from build123d import *

# Parameters (mm, degrees)
SKETCH1_R           = 15
BOSS_EXTRUDE1_DEPTH = 6
SKETCH2_R           = 30
BOSS_EXTRUDE2_DEPTH = 3
SKETCH5_R           = 10
CUT_EXTRUDE2_DEPTH  = 44.370496884
SKETCH8_R           = 2.5
CUT_EXTRUDE3_DEPTH  = 44.370496884


with BuildPart() as part:
    # Sketch1 → Boss-Extrude1 (new body)
    with BuildSketch(Plane.XY):
        Circle(SKETCH1_R)
    extrude(amount=BOSS_EXTRUDE1_DEPTH)

    # Sketch2 → Boss-Extrude2 (add)
    with BuildSketch(Plane.XY.offset(6)):
        Circle(SKETCH2_R)
    extrude(amount=BOSS_EXTRUDE2_DEPTH)

    # Sketch5 → Cut-Extrude2 (cut, through all)
    with BuildSketch(Plane(origin=(0, 0, 0), x_dir=(-1, 0, 0), z_dir=(0, 0, -1))):
        Circle(SKETCH5_R)
    extrude(amount=-CUT_EXTRUDE2_DEPTH, mode=Mode.SUBTRACT)

    # Sketch8 → Cut-Extrude3 (cut, through all)
    with BuildSketch(Plane.XY.offset(9)):
        with Locations((0, 25)):
            Circle(SKETCH8_R)
        with Locations((8.550503583, 23.49231552)):
            Circle(SKETCH8_R)
        with Locations((16.069690242, 19.151111078)):
            Circle(SKETCH8_R)
        with Locations((21.650635095, 12.5)):
            Circle(SKETCH8_R)
        with Locations((24.620193825, 4.341204442)):
            Circle(SKETCH8_R)
        with Locations((24.620193825, -4.341204442)):
            Circle(SKETCH8_R)
        with Locations((21.650635095, -12.5)):
            Circle(SKETCH8_R)
        with Locations((16.069690242, -19.151111078)):
            Circle(SKETCH8_R)
        with Locations((8.550503583, -23.49231552)):
            Circle(SKETCH8_R)
        with Locations((0, -25)):
            Circle(SKETCH8_R)
        with Locations((-8.550503583, -23.49231552)):
            Circle(SKETCH8_R)
        with Locations((-16.069690242, -19.151111078)):
            Circle(SKETCH8_R)
        with Locations((-21.650635095, -12.5)):
            Circle(SKETCH8_R)
        with Locations((-24.620193825, -4.341204442)):
            Circle(SKETCH8_R)
        with Locations((-24.620193825, 4.341204442)):
            Circle(SKETCH8_R)
        with Locations((-21.650635095, 12.5)):
            Circle(SKETCH8_R)
        with Locations((-16.069690242, 19.151111078)):
            Circle(SKETCH8_R)
        with Locations((-8.550503583, 23.49231552)):
            Circle(SKETCH8_R)
    extrude(amount=-CUT_EXTRUDE3_DEPTH, mode=Mode.SUBTRACT)


solid = part.part
Input: part model. Units: mm. Frame: model coordinates. A direction names the side the tool comes from. Give positions to 0.01 mm unless a question says otherwise; leave off trailing zeros. Loops run counter-clockwise (first coordinate to the right, second up) from the corner with the lowest first, then second, coordinate; pieces in that order, holes last. Notation, with made-up numbers: (-15.75, -28) -> (40.25, -28) arc R8 ccw to (40.25, -22) -> close; hole circle Ø6 at (45, 64.5). An arc over 180 degrees is marked (long way). Answer as a JSON object with one key per item and string values. Group by question number.
Item 1: Line query: probe 1 along X at (y, z) = (-20, 7.5); probe 2 along Y at (x, z) = (10.5, 8); probe 3 along Y at (x, z) = (0, 6.8). Output: solid intervals per line, ascending.
Item 2: Pin query (flat end, axial travel): P1, Ø5, axis at x = 10.5, z = 2.5, coming from the +Y side; P2, Ø4, axis at x = -24.62, y = -4.34, coming from the -Z side; P3, Ø6, axis at x = -8.55, y = 23.49, coming from the -Z side; P4, Ø1.5, axis at y = -12.5, z = 3.5, coming from the -X side. Return the tip coordinate at first contact, or that it passes through.
Item 3: Cut plane D-D, the plane z = 3.75. Return the cut outline in (x, y), and give its area (3 significant figures).
Item 4: Cut plane B-B, the plane y = 0. Return the cut outline in (x, z).
Item 5: Cut plane C-C, the plane x = -17.5. Return the cut outline in (y, z), and give its area (3 significant figures).
Item 6: Reachability of faces 4 (the cylindrical face through (-16.61, -21.59, 7.52)), 5 (the flat face through (6, 14, 6)) from +Z, -Z, +X, -X, +Y, -Y: full face, straight path, thin tool, end or side. Return the list, or none.
Item 7: Pull-direction query (Y, two-part tool) for faces 1 (the cylindrical face through (26.93, 3.38, 7.52)), 2 (the flat face through (13, 0, 9)), 3 (the cylindrical face through (-29.97, 1.32, 7.48)); classes: released by +Y, released by -Y, zero draft, split by the parting line, or undercut.
Item 8: Cut plane A-A, the plane x = 0. Return the cut outline in (y, z).
Checks:
{
 "1": {"probe 1": "x = -22.36 to -18.42, -13.72 to 13.72, 18.42 to 22.36", "probe 2": "y = -28.1 to -25.06, -21.93 to 21.93, 25.06 to 28.1", "probe 3": "y = -30 to -27.5, -22.5 to -10, 10 to 22.5, 27.5 to 30"},
 "2": {"P1": "stops at y = 12.69", "P2": "passes through", "P3": "stops at z = 6", "P4": "stops at x = -9.32"},
 "3": {"outline": "circle Ø30 at (0, 0); hole circle Ø20 at (0, 0)", "area": "393 mm²"},
 "4": {"outline": "(-30, 6) -> (-15, 6) -> (-15, 0) -> (-10, 0) -> (-10, 9) -> (-30, 9) -> close; (10, 0) -> (15, 0) -> (15, 6) -> (30, 6) -> (30, 9) -> (10, 9) -> close"},
 "5": {"outline": "(-24.37, 6) -> (-21.2, 6) -> (-21.2, 9) -> (-24.37, 9) -> close; (-17.1, 6) -> (17.1, 6) -> (17.1, 9) -> (-17.1, 9) -> close; (21.2, 6) -> (24.37, 6) -> (24.37, 9) -> (21.2, 9) -> close", "area": "122 mm²"},
 "6": {"face 4": "+Z, -Z", "face 5": "-Z"},
 "7": {"face 1": "undercut", "face 2": "zero draft", "face 3": "split by the parting line"},
 "8": {"outline": "(-30, 6) -> (-27.5, 6) -> (-27.5, 9) -> (-30, 9) -> close; (-22.5, 6) -> (-15, 6) -> (-15, 0) -> (-10, 0) -> (-10, 9) -> (-22.5, 9) -> close; (10, 0) -> (15, 0) -> (15, 6) -> (22.5, 6) -> (22.5, 9) -> (10, 9) -> close; (27.5, 6) -> (30, 6) -> (30, 9) -> (27.5, 9) -> close"}
}
